```python
from build123d import *

# Parameters (mm, degrees)
F0_R     = 2.05
F1_DEPTH = 50


with BuildPart() as f1:
    # F0 (on Top) → F1 (new body)
    with BuildSketch(Plane.XY):
        with BuildLine():
            ThreePointArc((7.5, 0), (0, 7.5), (-7.5, 0))
            Line((-7.5, 0), (-7.5, -6))
            Line((-7.5, -6), (7.5, -6))
            Line((7.5, -6), (7.5, 0))
        make_face()
        Circle(F0_R, mode=Mode.SUBTRACT)
    extrude(amount=F1_DEPTH)


solid = f1.part
```
CAD build for the part. Positions are in the model's coordinates, mm. Give positions to 0.01 mm unless a question says otherwise; leave off trailing zeros. Loops run counter-clockwise (first coordinate to the right, second up) from the corner with the lowest first, then second, coordinate; pieces in that order, holes last. Notation, with made-up numbers: (15, 21) -> (24, 21) arc R15 cw to (24, 41) -> close; hole circle Ø3 at (84.25, 46.25). An arc over 180 degrees is marked (long way). Use a Markdown table: item, result.
1. Slice it at B-B (z = 26). List the corners of the cut face in (x, y), plus the area to 3 significant figures.
Check result:
| item | result |
|---|---|
| outline | (-7.5, -6) -> (7.5, -6) -> (7.5, 0) arc R7.5 ccw to (-7.5, 0) -> close; hole circle Ø4.1 at (0, 0) |
| area | 165 mm^2 |
2. Slice it at C-C (y = 0.5). List the corners of the cut face in (x, z).
Check result:
| item | result |
|---|---|
| outline | (-7.48, 0) -> (-1.99, 0) -> (-1.99, 50) -> (-7.48, 50) -> close; (1.99, 0) -> (7.48, 0) -> (7.48, 50) -> (1.99, 50) -> close |
3. Flat gauge pins, fed straight in: pin 1 (8 mm diameter, centred on y = 0.5, z = 12.5, fed in from +X); pin 2 (4 mm diameter, centred on x = 5, z = 40.5, fed in from +Y). Where does each tip first touch, or does it go through?
Check result:
| item | result |
|---|---|
| pin 1 | stops at x = 7.5 |
| pin 2 | stops at y = 6.87 |
4. Wall check: L1, parallel to Y at x = 0, z = 15.5; L2, parallel to X at y = -0.25, z = 6; L3, parallel to Y at x = -1, z = 28. Give the ranges that are in metal, low to high. Write a range as [from, to].
Check result:
| item | result |
|---|---|
| L1 | y = [-6, -2.05], [2.05, 7.5] |
| L2 | x = [-7.5, -2.03], [2.03, 7.5] |
| L3 | y = [-6, -1.79], [1.79, 7.43] |
5. Mould opens along Y. For faces 1 (the flat face through (0, -6, 25)), 2 (the cylindrical face through (0.16, 7.5, 24.65)), 3 (the cylindrical face through (-0.267, 2.033, 24.65)), 4 (the flat face through (7.5, -3, 25)) say: pulls with the +Y half, pulls with the -Y half, needs draft (parallel to the pull), parting line crosses it, or undercut.
Check result:
| item | result |
|---|---|
| face 1 | pulls with the -Y half |
| face 2 | pulls with the +Y half |
| face 3 | undercut |
| face 4 | needs draft |
6. Slice it at A-A (x = 0). List the corners of the cut face in (y, z).
Check result:
| item | result |
|---|---|
| outline | (-6, 0) -> (-2.05, 0) -> (-2.05, 50) -> (-6, 50) -> close; (2.05, 0) -> (7.5, 0) -> (7.5, 50) -> (2.05, 50) -> close |
